```python
from build123d import *

# Parameters (mm, degrees)
BOX002_W                       = 161
BOX002_H                       = 2
BOX002_DEPTH                   = 15
BOX001_W                       = 163
BOX001_H                       = 2.5
BOX001_DEPTH                   = 17
BOX_W                          = 165
BOX_H                          = 6.5
BOX_DEPTH                      = 19
PART_MIRRORING_PLACEMENT_ANGLE = 180


with BuildPart() as cube002:
    # Box002 → Box002 (new body)
    with BuildSketch(Plane.XY.offset(4)):
        with Locations((80.5, 1)):
            Rectangle(BOX002_W, BOX002_H)
    extrude(amount=BOX002_DEPTH)


with BuildPart() as cube001:
    # Box001 → Box001 (new body)
    with BuildSketch(Plane(origin=(0, 2, 2), x_dir=(1, 0, 0), z_dir=(0, 0, 1))):
        with Locations((81.5, 1.25)):
            Rectangle(BOX001_W, BOX001_H)
    extrude(amount=BOX001_DEPTH)


with BuildPart() as cut001:
    # Box → Box (new body)
    with BuildSketch(Plane.XY):
        with Locations((82.5, 3.25)):
            Rectangle(BOX_W, BOX_H)
    extrude(amount=BOX_DEPTH)

    # Cut: cut Cube001
    add(cube001.part, mode=Mode.SUBTRACT)

    # Cut001: cut Cube002
    add(cube002.part, mode=Mode.SUBTRACT)


with BuildPart() as part_mirroring:
    # Part__Mirroring: instance of Cut001
    add(cut001.part.mirror(Plane(origin=(0, 0, 0), x_dir=(0, 1, 0), z_dir=(0, 0, 1))))


with BuildPart() as part_mirroring_1:
    # Part__Mirroring placement: moved
    add(part_mirroring.part.rotate(Axis((0, 0, 0), (0, 1, 0)), PART_MIRRORING_PLACEMENT_ANGLE))


solid = part_mirroring_1.part
```
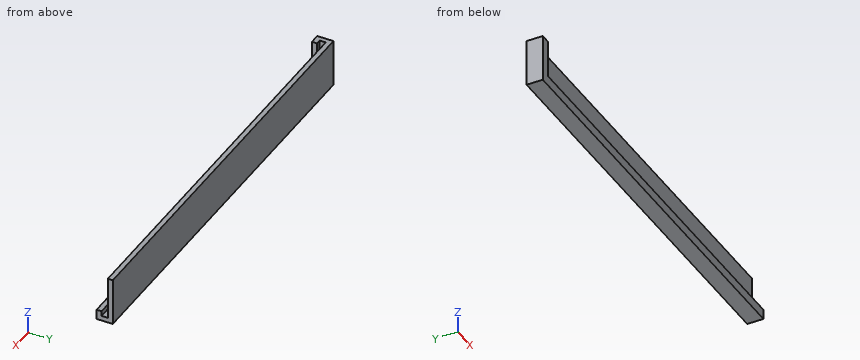
Verification items for the finished model (mm, model axes). Give positions to 0.01 mm unless a question says otherwise; leave off trailing zeros. Order: outer loops, then holes, each group sorted by start corner. A loop starts at its lowest first (then second) coordinate and runs counter-clockwise, first axis right, second up. Notation, with made-up numbers: M 38.5,6 L 49.5,6 A20 ccw 49.5,19 Z; hole C 71.25,-1 d4. An arc over 180 degrees is marked long. Return JSON: item names as keys, results as strings. Group by question number.
1) Section check B-B on z = 12.75. Record the cut outline in (x, y).
2) Section check A-A on x = -155. Record the cut outline in (y, z), and give its area (3 significant figures).
3) Go/stop test with flat-tipped pins: pin 1 Ø4 at (x, z) = (-21, 8) entering from -Y; pin 2 Ø0.6 at (x, y) = (-120, 0.5) entering from +Z; pin 3 Ø2 at (y, z) = (0.5, 9.5) entering from +X. Record where each tip stops, or that it passes through.
4) Scan lines: line 1 (Y direction, x = -67, z = 6.75); line 2 (X direction, y = 1.25, z = 9.5); line 3 (X direction, y = 2.25, z = 4.25). Record each from-to range of solid material in increasing order.
Answer block:
{
 "1": {"outline": "M -165,0 L -161,0 L -161,2 L -163,2 L -163,4.5 L 0,4.5 L 0,6.5 L -165,6.5 Z"},
 "2": {"outline": "M 0,0 L 6.5,0 L 6.5,19 L 4.5,19 L 4.5,2 L 2,2 L 2,4 L 0,4 Z", "area": "51.0 mm^2"},
 "3": {"pin 1": "stops at y = 4.5", "pin 2": "stops at z = 4", "pin 3": "stops at x = -161"},
 "4": {"line 1": "y = 4.5 to 6.5", "line 2": "x = -165 to -161", "line 3": "x = -165 to -163"}
}
